Here's how the part is built. I have some questions about the finished solid (model axes, mm). A direction names the side the tool comes from. Give positions to 0.01 mm unless a question says otherwise; leave off trailing zeros. Loops run counter-clockwise (first coordinate to the right, second up) from the corner with the lowest first, then second, coordinate; pieces in that order, holes last. Notation, with made-up numbers: (-3.75, 46.5) - (53.25, 46.5) arc R20 ccw to (53.25, 55.5) - close; hole circle Ø5 at (-14.5, -22.5). An arc over 180 degrees is marked (long way). Return JSON: item names as keys, results as strings. Group by question number.
(1) For P1, Ø20.5, axis at y = -41, z = 61.5, coming from the +X side; P2, Ø6, axis at x = 373, z = 165.5, coming from the +Y side; P3, Ø10, axis at x = 415, y = 36, coming from the +Z side; P4, Ø3, axis at x = 242, z = 106.5, coming from the -Y side, each with a flat end and sliding along its axis, tell me the tip position at first contact or that it passes through.
(2) If we section it at A-A (y = 76): Please give me the cut outline in (x, z), then the cut area to 3 significant figures.
(3) I need wall thicknesses on probe 1 along Z at (x, y) = (61.5, -41); probe 2 along X at (y, z) = (111.5, 45); probe 3 along Y at (x, z) = (174, 213). Which ranges of each line are inside material? Lowest first, please. Write a range as [from, to].
(4) If we section it at C-C (x = 140.5): Please give me the cut outline in (y, z).
(5) If we mould it in two halves opening along X, with no side actions, what happens to faces 1 (the flat face through (0, -13, 114)), 2 (the flat face through (245, -38, 99.62)), 3 (the flat face through (450.697, -38, 63))? For each: released by +X, released by -X, zero draft, split by the parting line, or undercut.
(6) If we section it at B-B (x = 429.5): Please give me the cut outline in (y, z).
(7) On a 3-axis mill with a long thin cutter (end or side, diameter ignored), from which of +Z, -Z, +X, -X, +Y, -Y can I reach the whole of each face in a straight line? I mean faces 4 (the flat face through (134.1, 75, 25)), 5 (the flat face through (273, -13, 122.073)), 6 (the flat face through (380, 75, 50.779)), 7 (the flat face through (80.19, 75, 25)). Say none if no direction works.
(8) If we section it at D-D (z = 68): Please give me the cut outline in (x, y).
```python
from build123d import *

# Parameters (mm, degrees)
F0_W     = 483.521879
F0_H     = 232.050955
F1_DEPTH = 25.4
F2_W     = 52.622199
F2_H     = 50.77935
F2_W_2   = 53.910152
F3_DEPTH = 152.4
F4_R     = 6.942146
F4_R_2   = 7.233065
F4_R_3   = 6.827798
F4_R_4   = 6.825473
F4_R_5   = 6.970363
F4_R_6   = 7.019906
F4_R_7   = 7.160675
F4_R_8   = 6.922756
F4_R_9   = 7.679718
F4_R_10  = 6.87136
F4_W     = 33.581532
F4_H     = 12.216136
F4_W_2   = 34.816921
F4_W_3   = 31.48967
F4_W_4   = 34.290463
F4_W_5   = 34.827173
F5_DEPTH = 25.4
F6_DEPTH = 25.4


with BuildPart() as f1:
    # F0 (on Front) → F1 (new body)
    with BuildSketch(Plane.XZ):
        with Locations((241.760939, 116.025477)):
            Rectangle(F0_W, F0_H)
    extrude(amount=F1_DEPTH)

    # F2 (on face) → F3 (join)
    with BuildSketch(Plane(origin=(0, 0, 0), x_dir=(-1, 0, 0), z_dir=(0, 1, 0))):
        with Locations((-379.599809, 25.389675)):
            Rectangle(F2_W, F2_H)
        with Locations((-107.145153, 25.389675)):
            Rectangle(F2_W_2, F2_H)
    extrude(amount=F3_DEPTH)

    # F4 (on face) → F5 (cut)
    with BuildSketch(Plane.XZ.offset(25.4)):
        with Locations((442.921937, 182.266369)):
            Circle(F4_R)
        with Locations((396.795809, 182.266369)):
            Circle(F4_R_2)
        with Locations((350.143939, 182.266369)):
            Circle(F4_R_3)
        with Locations((303.674549, 182.266369)):
            Circle(F4_R_4)
        with Locations((257.422805, 182.266369)):
            Circle(F4_R_5)
        with Locations((210.462064, 182.266369)):
            Circle(F4_R_6)
        with Locations((164.519146, 182.266369)):
            Circle(F4_R_7)
        with Locations((118.084826, 182.266369)):
            Circle(F4_R_8)
        with Locations((72.942153, 182.266369)):
            Circle(F4_R_9)
        with Locations((32.544691, 182.266369)):
            Circle(F4_R_10)
        with Locations((89.732919, 128.181107)):
            Rectangle(F4_W, F4_H)
        with Locations((181.927606, 128.181107)):
            Rectangle(F4_W_2, F4_H)
        with Locations((273.16764, 128.181107)):
            Rectangle(F4_W_3, F4_H)
        with Locations((367.28917, 128.181107)):
            Rectangle(F4_W_4, F4_H)
        with Locations((437.272459, 128.181107)):
            Rectangle(F4_W_5, F4_H)
    extrude(amount=-F5_DEPTH, mode=Mode.SUBTRACT)

    # F4 (on face) → F6 (join)
    with BuildSketch(Plane.XZ.offset(25.4)):
        Polygon((32.544691, 39.454777), (32.544691, 86.642593), (16.272346, 86.642593), (16.272346, 26.111573), (467.10965, 26.111573), (467.10965, 86.642593), (450.697422, 86.642593), (450.697422, 39.454777), align=None)
        Polygon((16.272346, 86.642593), (32.544691, 86.642593), (450.697422, 86.642593), (467.10965, 86.642593), (467.10965, 99.620059), (16.272346, 99.620059), align=None)
    extrude(amount=F6_DEPTH)


solid = f1.part
```
Values:
{
 "1": {"P1": "x = 467.11", "P2": "y = 0", "P3": "through", "P4": "y = -25.4"},
 "2": {"outline": "(80.19, 0) - (134.1, 0) - (134.1, 50.78) - (80.19, 50.78) - close; (353.29, 0) - (405.91, 0) - (405.91, 50.78) - (353.29, 50.78) - close", "area": "5,410 mm2"},
 "3": {"probe 1": "[26.11, 39.45], [86.64, 99.62]", "probe 2": "[80.19, 134.1], [353.29, 405.91]", "probe 3": "[-25.4, 0]"},
 "4": {"outline": "(-50.8, 26.11) - (-25.4, 26.11) - (-25.4, 0) - (0, 0) - (0, 232.05) - (-25.4, 232.05) - (-25.4, 99.62) - (-50.8, 99.62) - (-50.8, 86.64) - (-25.4, 86.64) - (-25.4, 39.45) - (-50.8, 39.45) - close"},
 "5": {"face 1": "released by -X", "face 2": "zero draft", "face 3": "undercut"},
 "6": {"outline": "(-50.8, 26.11) - (-25.4, 26.11) - (-25.4, 0) - (0, 0) - (0, 122.07) - (-25.4, 122.07) - (-25.4, 99.62) - (-50.8, 99.62) - (-50.8, 86.64) - (-25.4, 86.64) - (-25.4, 39.45) - (-50.8, 39.45) - close; (-25.4, 134.29) - (0, 134.29) - (0, 232.05) - (-25.4, 232.05) - close"},
 "7": {"face 4": "+Z, -Z, +Y", "face 5": "+Y, -Y", "face 6": "+Z, +X, -X, +Y", "face 7": "+Z, -Z, -X, +Y"},
 "8": {"outline": "(0, -25.4) - (16.27, -25.4) - (16.27, -50.8) - (32.54, -50.8) - (32.54, -25.4) - (450.7, -25.4) - (450.7, -50.8) - (467.11, -50.8) - (467.11, -25.4) - (483.52, -25.4) - (483.52, 0) - (0, 0) - close"}
}
